Read the model definition and answer for the solid it produces. Units are mm, in the model's axes. A direction names the side the tool comes from. Give positions to 0.01 mm unless a question says otherwise; leave off trailing zeros. Write each loop counter-clockwise with the first axis right and the second up, starting at its lowest first coordinate (ties: lowest second). Pieces come first, ordered by that corner, then holes. Notation, with made-up numbers: (41.5, -37.5) - (69.5, -37.5) arc R12 cw to (69.5, -28.5) - close; hole circle Ø9 at (75, 55). An arc over 180 degrees is marked (long way). Answer as a JSON object with one key per item and string values. Group by question number.
```python
from build123d import *

# Parameters (mm, degrees)
CUT_EXTRUDE1_DEPTH               = 18.915104549
F_3_8_18_NPSM_TAPPED_HOLE1_D     = 15.3162
F_3_8_18_NPSM_TAPPED_HOLE1_DEPTH = 9.525
F_3_8_18_NPSM_TAPPED_HOLE1_TIP   = 4.601450707


with BuildPart() as part:
    # Sketch1 → Revolve1 (revolve)
    with BuildSketch(Plane.XY, mode=Mode.PRIVATE) as revolve1_sk:
        Polygon((0, 9.525), (12.7, 9.525), (12.7, 0), (0.889, 0), (0.889, 8.255), (0, 8.255), align=None)
    revolve(revolve1_sk.sketch.rotate(Axis((0, 0, 0), (1, 0, 0)), 90), axis=Axis((0, 0, 0), (1, 0, 0)))

    # Sketch2 → Cut-Extrude1 (cut, through all)
    with BuildSketch(Plane.ZY.offset(-0.889)):
        with BuildLine():
            Line((-4.7625, -2.54), (-4.7625, 2.54))
            ThreePointArc((-4.7625, 2.54), (0, 7.3025), (4.7625, 2.54))
            Line((4.7625, 2.54), (4.7625, -2.54))
            ThreePointArc((4.7625, -2.54), (0, -7.3025), (-4.7625, -2.54))
        make_face()
    extrude(amount=-CUT_EXTRUDE1_DEPTH, mode=Mode.SUBTRACT)

    # 3/8-18 NPSM Tapped Hole1
    with Locations(Plane(origin=(12.7, 0, 0), x_dir=(0, 0, -1), z_dir=(1, 0, 0))):
        with Locations((0, 0)):
            Hole(F_3_8_18_NPSM_TAPPED_HOLE1_D / 2, depth=F_3_8_18_NPSM_TAPPED_HOLE1_DEPTH)
            with Locations((0, 0, -(F_3_8_18_NPSM_TAPPED_HOLE1_DEPTH + F_3_8_18_NPSM_TAPPED_HOLE1_TIP / 2))):  # 118° drill point
                Cone(0, F_3_8_18_NPSM_TAPPED_HOLE1_D / 2, F_3_8_18_NPSM_TAPPED_HOLE1_TIP, mode=Mode.SUBTRACT)


solid = part.part
```
1) Find the intervals of material crossed by line 1 (Y direction, x = 0.4, z = 0) (3 decimals); line 2 (Y direction, x = 11.75, z = 0.25); line 3 (Z direction, x = 5.5, y = 6.75), in increasing order. Write a range as [from, to].
2) Flat-ended cylindrical pins translate along their axes: pin 1 Ø1 at (x, y) = (1.5, 1) entering from +Z; pin 2 Ø5 at (y, z) = (-1.5, -3) entering from -X. Find the tip coordinate at first contact, or state that the pin passes through.
3) Which of the six approach directions +Z, -Z, +X, -X, +Y, -Y give full straight-line access (tool end or side, diameter ignored) to faces 4 (the cylindrical face through (7.87, 0.34, -7.65)), 5 (the cylindrical face through (0.438, 7.324, 3.809)), 6 (the flat face through (12.7, -8, 1)), 7 (the flat face through (1.2, 0, 4.762))?
4) Find section B-B, the plane z = 0. Write down the section's boundary in (x, y) (1 decimal).
5) Find section A-A, the plane y = 0. Write down the section's boundary in (x, z) (1 decimal), and give its area (3 significant figures).
6) Find section C-C, the plane x = 6.25. Write down the section's boundary in (y, z) (3 decimals), and give its area (3 significant figures).
7) For a pull along Z with two mould halves and no side action, classify faces 1 (the cylindrical face through (1.7, -7.3, 0.1)), 2 (the flat face through (0, -8, 3)), 3 (the cylindrical face through (6.44, 9.3, -2.06)) as released by +Z, released by -Z, zero draft, split by the parting line, or undercut.
Values follow:
{
 "1": {"line 1": "y = [-9.525, -8.255], [8.255, 9.525]", "line 2": "y = [-9.52, -7.65], [7.65, 9.52]", "line 3": "z = [-6.72, -3.62], [3.62, 6.72]"},
 "2": {"pin 1": "stops at z = 9.51", "pin 2": "stops at x = 0.89"},
 "3": {"face 4": "+X", "face 5": "-X", "face 6": "+Z, -Z, +X, +Y, -Y", "face 7": "+X, -X"},
 "4": {"outline": "(0, -9.5) - (12.7, -9.5) - (12.7, -7.7) - (3.2, -7.7) - (3, -7.3) - (0.9, -7.3) - (0.9, -8.3) - (0, -8.3) - close; (0, 8.3) - (0.9, 8.3) - (0.9, 7.3) - (3, 7.3) - (3.2, 7.7) - (12.7, 7.7) - (12.7, 9.5) - (0, 9.5) - close"},
 "5": {"outline": "(0, -9.5) - (12.7, -9.5) - (12.7, -7.7) - (3.2, -7.7) - (1.4, -4.8) - (0.9, -4.8) - (0.9, -8.3) - (0, -8.3) - close; (0, 8.3) - (0.9, 8.3) - (0.9, 4.8) - (1.4, 4.8) - (3.2, 7.7) - (12.7, 7.7) - (12.7, 9.5) - (0, 9.5) - close", "area": "54.6 mm2"},
 "6": {"outline": "circle Ø19.05 at (0, 0); hole circle Ø15.316 at (0, 0)", "area": "101 mm2"},
 "7": {"face 1": "undercut", "face 2": "zero draft", "face 3": "split by the parting line"}
}
